Check sheet for the modelled part. Datum: model origin and axes. Units: mm. Face numbers are marked on the shaded views. A direction names the side the tool comes from. Round coordinates to 2 decimals unless told otherwise and drop trailing zeros.
Q1. Mould release check, pull along X, two halves, no side actions. Record for the marked faces 4, 5 and 6: +X half, -X half, draft (parallel to the pull), parting line (faces both ways), or undercut.
Q2. Set-up check for the marked faces 1, 2 and 3: record each of +Z, -Z, +X, -X, +Y, -Y from which the full face is reachable in a straight line by a thin tool's end or side.
Q3. Depth check by flat-ended pin: P1, Ø2, axis at x = -110, z = -51.5, coming from the -Y side; P2, Ø2, axis at x = 493.5, z = -193.5, coming from the +Y side; P3, Ø1.5, axis at x = 95.5, y = 116.5, coming from the -Z side. Enter the tip coordinate at first touch or a pass-through.
Q4. Scan lines: probe 1 along Z at (x, y) = (-200, 157); probe 2 along X at (y, z) = (7, -81.5); probe 3 along Y at (x, z) = (480.5, 195.5). Record each from-to range of solid material in increasing order.
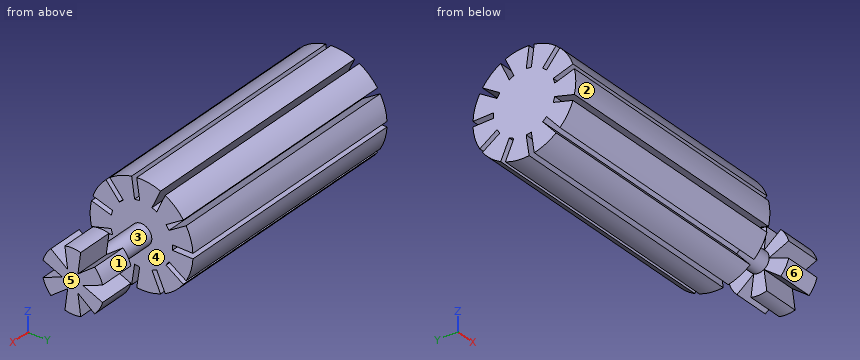
Autodesk Inventor part; units mm, degrees
ref_plane "YZ Plane" through (0, 0, 0) normal (1, 0, 0) x (0, 1, 0)
ref_plane "XZ Plane" through (0, 0, 0) normal (0, 1, 0) x (-1, 0, 0)
ref_plane "XY Plane" through (0, 0, 0) normal (0, 0, 1) x (1, 0, 0)
sketch "Sketch1" plane through (0, 0, 0) normal (1, 0, 0) x (0, 1, 0)
  line L0 (253.6823, 12.7) -> (152.4, 12.7)
  line L1 (152.4, 12.7) -> (152.4, -12.7)
  line L2 (152.4, -12.7) -> (253.6823, -12.7)
  line L3 (228.6, 0) -> (152.4, 0) construction
  line L4 (206.545, 147.8349) -> (121.3409, 93.0776)
  line L5 (121.3409, 93.0776) -> (135.0732, 71.7097)
  line L6 (135.0732, 71.7097) -> (220.2773, 126.4671)
  line L7 (93.8311, 236.0333) -> (51.7569, 143.9037)
  line L8 (51.7569, 143.9037) -> (74.8616, 133.3521)
  line L9 (74.8616, 133.3521) -> (116.9358, 225.4818)
  line L10 (-48.6735, 249.2928) -> (-34.2595, 149.0414)
  line L11 (-34.2595, 149.0414) -> (-9.118, 152.6562)
  line L12 (-9.118, 152.6562) -> (-23.532, 252.9076)
  line L13 (-175.7246, 183.4036) -> (-109.3988, 106.8595)
  line L14 (-109.3988, 106.8595) -> (-90.2028, 123.493)
  line L15 (-90.2028, 123.493) -> (-156.5286, 200.037)
  line L16 (-246.9844, 59.285) -> (-149.8047, 30.7505)
  line L17 (-149.8047, 30.7505) -> (-142.6487, 55.1216)
  line L18 (-142.6487, 55.1216) -> (-239.8284, 83.6561)
  line L19 (-239.8284, -83.6561) -> (-142.6487, -55.1216)
  line L20 (-142.6487, -55.1216) -> (-149.8047, -30.7505)
  line L21 (-149.8047, -30.7505) -> (-246.9844, -59.285)
  line L22 (-156.5286, -200.037) -> (-90.2028, -123.493)
  line L23 (-90.2028, -123.493) -> (-109.3988, -106.8595)
  line L24 (-109.3988, -106.8595) -> (-175.7246, -183.4036)
  line L25 (-23.532, -252.9076) -> (-9.118, -152.6562)
  line L26 (-9.118, -152.6562) -> (-34.2595, -149.0414)
  line L27 (-34.2595, -149.0414) -> (-48.6735, -249.2928)
  line L28 (116.9358, -225.4818) -> (74.8616, -133.3521)
  line L29 (74.8616, -133.3521) -> (51.7569, -143.9037)
  line L30 (51.7569, -143.9037) -> (93.8311, -236.0333)
  line L31 (220.2773, -126.4671) -> (135.0732, -71.7097)
  line L32 (135.0732, -71.7097) -> (121.3409, -93.0776)
  line L33 (121.3409, -93.0776) -> (206.545, -147.8349)
  arc A0 (253.6823, 12.7) -> (220.2773, 126.4671) centre (0, 0) ccw
  arc A1 (220.2773, -126.4671) -> (253.6823, -12.7) centre (0, 0) ccw
  arc A2 (116.9358, -225.4818) -> (206.545, -147.8349) centre (0, 0) ccw
  arc A3 (-23.532, -252.9076) -> (93.8311, -236.0333) centre (0, 0) ccw
  arc A4 (-156.5286, -200.037) -> (-48.6735, -249.2928) centre (0, 0) ccw
  arc A5 (-239.8284, -83.6561) -> (-175.7246, -183.4036) centre (0, 0) ccw
  arc A6 (-246.9844, 59.285) -> (-246.9844, -59.285) centre (0, 0) ccw
  arc A7 (-175.7246, 183.4036) -> (-239.8284, 83.6561) centre (0, 0) ccw
  arc A8 (-48.6735, 249.2928) -> (-156.5286, 200.037) centre (0, 0) ccw
  arc A9 (206.545, 147.8349) -> (116.9358, 225.4818) centre (0, 0) ccw
  arc A10 (93.8311, 236.0333) -> (-23.532, 252.9076) centre (0, 0) ccw
  point P0 (128.207, 82.3937)
  point P1 (63.3092, 138.6279)
  point P2 (-21.6888, 150.8488)
  point P3 (-99.8008, 115.1762)
  point P4 (-146.2267, 42.936)
  point P5 (-146.2267, -42.936)
  point P6 (-99.8008, -115.1762)
  point P7 (-21.6888, -150.8488)
  point P8 (63.3092, -138.6279)
  point P9 (128.207, -82.3937)
  dimension "d4" = 254
  dimension "d5" = 152.4
  dimension "d6" = 25.4
extrude "Extrusion1" add sketch "Sketch1" along normal mid plane 1219.2
sketch "Sketch2" plane through (0, 0, 0) normal (0, 0, 1) x (1, 0, 0)
  line L0 (609.6, 0) -> (1041.4, 0)
  line L1 (1041.4, 0) -> (1041.4, 152.4)
  line L2 (1041.4, 152.4) -> (863.6, 152.4)
  line L3 (863.6, 152.4) -> (863.6, 50.8)
  line L4 (863.6, 50.8) -> (609.6, 50.8)
  line L5 (609.6, -23.532) -> (609.6, 93.8311)
  point P0 (0, 0)
  dimension "d9" = 101.6
  dimension "d10" = 177.8
  dimension "d11" = 304.8
  dimension "d12" = 254
revolve "Revolution1" add sketch "Sketch2" angle 360 about axis through (609.6, 0, 0) along (1, 0, 0)
sketch "Sketch3" plane through (1041.4, 0, 0) normal (1, 0, 0) x (0, 0, -1)
  circle A0 centre (0, 0) radius 152.4 construction
  circle A1 centre (0, 0) radius 152.4 construction
  line L0 (-39.884, 147.0885) -> (0, 50.8)
  line L1 (0, 50.8) -> (39.884, 147.0885)
  line L2 (0, 0) -> (0, 152.4) construction
  line L3 (-43.9941, 25.4) -> (-107.4404, 108.0848)
  line L4 (-147.3244, 39.0037) -> (-43.9941, 25.4)
  line L5 (-43.9941, -25.4) -> (-147.3244, -39.0037)
  line L6 (-107.4404, -108.0848) -> (-43.9941, -25.4)
  line L7 (0, -50.8) -> (-39.884, -147.0885)
  line L8 (39.884, -147.0885) -> (0, -50.8)
  line L9 (43.9941, -25.4) -> (107.4404, -108.0848)
  line L10 (147.3244, -39.0037) -> (43.9941, -25.4)
  line L11 (43.9941, 25.4) -> (147.3244, 39.0037)
  line L12 (107.4404, 108.0848) -> (43.9941, 25.4)
  arc A2 (39.884, 147.0885) -> (-39.884, 147.0885) centre (0, 0) ccw
  arc A3 (147.3244, 39.0037) -> (107.4404, 108.0848) centre (0, 0) ccw
  arc A4 (107.4404, -108.0848) -> (147.3244, -39.0037) centre (0, 0) ccw
  arc A5 (-39.884, -147.0885) -> (39.884, -147.0885) centre (0, 0) ccw
  arc A6 (-107.4404, 108.0848) -> (-147.3244, 39.0037) centre (0, 0) ccw
  arc A7 (-147.3244, -39.0037) -> (-107.4404, -108.0848) centre (0, 0) ccw
  dimension "d14" = 50.8
  dimension "d15" = 45
  dimension "d18" = 360
extrude "Extrusion2" cut sketch "Sketch3" against normal up to surface (177.8 mm away)
properties part number "Hydraulic ShaftCJE" material "Steel, High Strength, Low Alloy"
Results found:
1. face 4: undercut
1. face 5: +X half
1. face 6: draft
2. face 1: +Z, +X, +Y
2. face 2: +X, -X, -Y
2. face 3: none
3. P1: stops at y = -248.93
3. P2: stops at y = 165.71
3. P3: stops at z = -225.48
4. probe 1: z = -199.67 to -115.99, -85.8 to -12.7, 12.7 to 85.8, 115.99 to 199.67
4. probe 2: x = -609.6 to 609.6, 863.6 to 1041.4
4. probe 3: y = -152.6 to -40.94, -15.28 to 75.32, 103.24 to 162.16
